```python
from build123d import *

# Parameters (mm, degrees)
BASE_EXTRUDE_DEPTH  = 12.7
BOSS_EXTRUDE1_DEPTH = 12.7


with BuildPart() as part:
    # Sketch1 → Base-Extrude (new, symmetric)
    with BuildSketch(Plane.XY):
        with BuildLine():
            Line((-20.6375, 19.1389), (-20.6375, 11.29515134))
            ThreePointArc((-20.6375, 11.29515134), (-19.1389, 8.6995), (-20.6375, 6.10384866))
            Line((-20.6375, 6.10384866), (-20.6375, 1.4986))
            ThreePointArc((-20.6375, 1.4986), (-20.198570222, 0.438929778), (-19.1389, 0))
            Line((-19.1389, 0), (19.1389, 0))
            ThreePointArc((19.1389, 0), (20.198570222, 0.438929778), (20.6375, 1.4986))
            Line((20.6375, 1.4986), (20.6375, 6.10384866))
            ThreePointArc((20.6375, 6.10384866), (19.1389, 8.6995), (20.6375, 11.29515134))
            Line((20.6375, 11.29515134), (20.6375, 19.1389))
            ThreePointArc((20.6375, 19.1389), (20.198570222, 20.198570222), (19.1389, 20.6375))
            Line((19.1389, 20.6375), (12.6111, 20.6375))
            ThreePointArc((12.6111, 20.6375), (11.551429778, 20.198570222), (11.1125, 19.1389))
            Line((11.1125, 19.1389), (11.1125, 14.2875))
            Line((11.1125, 14.2875), (12.6111, 14.2875))
            Line((12.6111, 14.2875), (12.6111, 19.1389))
            Line((12.6111, 19.1389), (19.1389, 19.1389))
            Line((19.1389, 19.1389), (19.1389, 12.050471471))
            ThreePointArc((19.1389, 12.050471471), (17.6403, 8.6995), (19.1389, 5.348528529))
            Line((19.1389, 5.348528529), (19.1389, 1.4986))
            Line((19.1389, 1.4986), (-19.1389, 1.4986))
            Line((-19.1389, 1.4986), (-19.1389, 5.348528529))
            ThreePointArc((-19.1389, 5.348528529), (-17.6403, 8.6995), (-19.1389, 12.050471471))
            Line((-19.1389, 12.050471471), (-19.1389, 19.1389))
            Line((-19.1389, 19.1389), (-12.6111, 19.1389))
            Line((-12.6111, 19.1389), (-12.6111, 14.2875))
            Line((-12.6111, 14.2875), (-11.1125, 14.2875))
            Line((-11.1125, 14.2875), (-11.1125, 19.1389))
            ThreePointArc((-11.1125, 19.1389), (-11.551429778, 20.198570222), (-12.6111, 20.6375))
            Line((-12.6111, 20.6375), (-19.1389, 20.6375))
            ThreePointArc((-19.1389, 20.6375), (-20.198570222, 20.198570222), (-20.6375, 19.1389))
        make_face()
    base_extrude = extrude(amount=BASE_EXTRUDE_DEPTH, both=True)

    # Mirror1: Base-Extrude across plane
    add(base_extrude.mirror(Plane.ZX))

    # Sketch2 → Boss-Extrude1 (add, symmetric)
    with BuildSketch(Plane(origin=(20.16125, 0.15875, 0), x_dir=(0, -1, 0), z_dir=(0, 0, 1))):
        with BuildLine():
            Line((-20.47875, 19.61515), (-20.47875, 11.77140134))
            ThreePointArc((-20.47875, 11.77140134), (-18.98015, 9.17575), (-20.47875, 6.58009866))
            Line((-20.47875, 6.58009866), (-20.47875, 1.97485))
            ThreePointArc((-20.47875, 1.97485), (-20.039820222, 0.915179778), (-18.98015, 0.47625))
            Line((-18.98015, 0.47625), (19.29765, 0.47625))
            ThreePointArc((19.29765, 0.47625), (20.357320222, 0.915179778), (20.79625, 1.97485))
            Line((20.79625, 1.97485), (20.79625, 6.58009866))
            ThreePointArc((20.79625, 6.58009866), (19.29765, 9.17575), (20.79625, 11.77140134))
            Line((20.79625, 11.77140134), (20.79625, 19.61515))
            ThreePointArc((20.79625, 19.61515), (20.357320222, 20.674820222), (19.29765, 21.11375))
            Line((19.29765, 21.11375), (12.76985, 21.11375))
            ThreePointArc((12.76985, 21.11375), (11.710179778, 20.674820222), (11.27125, 19.61515))
            Line((11.27125, 19.61515), (11.27125, 14.76375))
            Line((11.27125, 14.76375), (12.76985, 14.76375))
            Line((12.76985, 14.76375), (12.76985, 19.61515))
            Line((12.76985, 19.61515), (19.29765, 19.61515))
            Line((19.29765, 19.61515), (19.29765, 12.526721471))
            ThreePointArc((19.29765, 12.526721471), (17.79905, 9.17575), (19.29765, 5.824778529))
            Line((19.29765, 5.824778529), (19.29765, 1.97485))
            Line((19.29765, 1.97485), (-18.98015, 1.97485))
            Line((-18.98015, 1.97485), (-18.98015, 5.824778529))
            ThreePointArc((-18.98015, 5.824778529), (-17.48155, 9.17575), (-18.98015, 12.526721471))
            Line((-18.98015, 12.526721471), (-18.98015, 19.61515))
            Line((-18.98015, 19.61515), (-12.45235, 19.61515))
            Line((-12.45235, 19.61515), (-12.45235, 14.76375))
            Line((-12.45235, 14.76375), (-10.95375, 14.76375))
            Line((-10.95375, 14.76375), (-10.95375, 19.61515))
            ThreePointArc((-10.95375, 19.61515), (-11.392679778, 20.674820222), (-12.45235, 21.11375))
            Line((-12.45235, 21.11375), (-18.98015, 21.11375))
            ThreePointArc((-18.98015, 21.11375), (-20.039820222, 20.674820222), (-20.47875, 19.61515))
        make_face()
    extrude(amount=BOSS_EXTRUDE1_DEPTH, both=True)


solid = part.part
```
The listing builds one solid part. Answer for the finished solid, in the listing's coordinates (mm). A direction names the side the tool comes from. Give positions to 0.01 mm unless a question says otherwise; leave off trailing zeros. Write each loop counter-clockwise with the first axis right and the second up, starting at its lowest first coordinate (ties: lowest second). Pieces come first, ordered by that corner, then holes. Notation, with made-up numbers: M -24,-29 L 13,-29 A36 cw 13,9 Z; hole C 72,-5.5 d6. An arc over 180 degrees is marked long. Write each question's results on one line, items separated by ' | '.
Q1. Consider L1, parallel to X at y = 15, z = -9.5 (1 decimal); L2, parallel to Y at x = 35, z = -11.5; L3, parallel to Y at x = -17.5, z = 2. Determine where each line is inside the solid, lowest interval first. Write a range as from..to.
Output values:
L1: -20.6..-19.1, -12.6..-11.1, 11.1..12.6, 19.1..22.1, 39.8..41.3 | L2: -20.64..-19.14, -12.61..-11.11, 11.11..12.61, 19.14..20.64 | L3: -20.64..-19.14, -1.5..1.5, 19.14..20.64
Q2. A tool of negligible diameter and unlimited length cuts with its end or side. For faces 3 (the flat face through (34.925, -12, 0)), 4 (the flat face through (-11.112, -17, 0)), 5 (the flat face through (-11.112, 17, 0)), from which of +Z, -Z, +X, -X, +Y, -Y can it reach the whole face along a straight path? Write none if from no direction.
Output values:
face 3: +Z, -Z | face 4: +Z, -Z, -Y | face 5: +Z, -Z, +Y
Q3. Section C-C, the plane x = 31 is taken. Write down the section's boundary in (y, z), then the cut area to 3 significant figures.
Output values:
outline: M -19.64,-12.7 L -17.96,-12.7 L -17.96,12.7 L -19.64,12.7 Z; M 17.96,-12.7 L 19.64,-12.7 L 19.64,12.7 L 17.96,12.7 Z | area: 85.5 mm2
Q4. Section A-A, the plane x = 14 is taken. Write down the section's boundary in (y, z), then the cut area to 3 significant figures.
Output values:
outline: M -20.64,-12.7 L -19.14,-12.7 L -19.14,12.7 L -20.64,12.7 Z; M -1.5,-12.7 L 1.5,-12.7 L 1.5,12.7 L -1.5,12.7 Z; M 19.14,-12.7 L 20.64,-12.7 L 20.64,12.7 L 19.14,12.7 Z | area: 152 mm2
Q5. Section B-B, the plane y = -16 is taken. Write down the section's boundary in (x, z) (1 decimal), then the cut area to 3 significant figures.
Output values:
outline: M -20.6,-12.7 L -19.1,-12.7 L -19.1,12.7 L -20.6,12.7 Z; M -12.6,-12.7 L -11.1,-12.7 L -11.1,12.7 L -12.6,12.7 Z; M 11.1,-12.7 L 12.6,-12.7 L 12.6,12.7 L 11.1,12.7 Z; M 19.1,-12.7 L 22.1,-12.7 L 22.1,12.7 L 19.1,12.7 Z; M 39.8,-12.7 L 41.3,-12.7 L 41.3,12.7 L 39.8,12.7 Z | area: 228 mm2
Q6. For a pull along X with two mould halves and no side action, classify faces 1 (the flat face through (37, -11.112, 0)), 2 (the flat face through (-16, -19.139, 0)) as released by +X, released by -X, zero draft, split by the parting line, or undercut.
Output values:
face 1: zero draft | face 2: undercut
Q7. Flat-ended cylindrical pins translate along their axes: P1, Ø4, axis at x = -11.5, y = -12, coming from the +Z side; P2, Ø1.2, axis at x = 11.5, z = -4.5, coming from the -Y side; P3, Ø10, axis at x = 1.5, z = 5.5, coming from the +Y side; P4, Ø3, axis at x = -3, z = -7.5, coming from the -Y side. Find the tip coordinate at first contact, or state that the pin passes through.
Output values:
P1: through | P2: y = -20.55 | P3: y = 1.5 | P4: y = -1.5
Q8. Section D-D, the plane y = 7.5 is taken. Write down the section's boundary in (x, z).
Output values:
outline: M -19.39,-12.7 L -17.8,-12.7 L -17.8,12.7 L -19.39,12.7 Z; M 17.8,-12.7 L 19.39,-12.7 L 19.39,12.7 L 17.8,12.7 Z; M 20.64,-12.7 L 22.14,-12.7 L 22.14,12.7 L 20.64,12.7 Z
